from build123d import *

# Parameters (mm, degrees)
OUTER_START                              = 2.286
OUTER_CLAMP_LATCH_CUT_EXTRUDE5_DEPTH     = 2.794
OUTER_START_2                            = -1.143
OUTER_CLAMP_LATCH_CUT_EXTRUDE5_2_DEPTH   = 2.4129999
OUTER_START_3                            = -0.508
OUTER_CLAMP_LATCH_CUT_EXTRUDE5_3_OUTLI_R = 0.79375
OUTER_CLAMP_LATCH_CUT_EXTRUDE5_3_DEPTH   = 1.651
OUTER_START_4                            = 3.429
OUTER_CLAMP_LATCH_CUT_EXTRUDE5_4_OUTLI_R = 0.79375
OUTER_CLAMP_LATCH_CUT_EXTRUDE5_4_DEPTH   = 1.651
OUTER_START_5                            = 5.08
OUTER_CLAMP_LATCH_CUT_EXTRUDE5_5_DEPTH   = 1.27
OUTER_START_6                            = 1.2699999
OUTER_CLAMP_LATCH_CUT_EXTRUDE5_6_DEPTH   = 1.0160001
OUTER_START_7                            = -5.207
OUTER_CLAMP_LATCH_CUT_EXTRUDE5_7_OUTLI_R = 0.508
OUTER_CLAMP_LATCH_CUT_EXTRUDE5_7_DEPTH   = 2.54
SKETCH1_W                                = 0.762
SKETCH1_H                                = 1.524
CUT_EXTRUDE1_DEPTH                       = 14.441616644


with BuildPart() as part:
    # <Outer Clamp Latch>-<Cut-Extrude5>: read off the stored shape, not the designer's step
    # <Outer Clamp Latch>-<Cut-Extrude5> outline → <Outer Clamp Latch>-<Cut-Extrude5> (new body)
    with BuildSketch(Plane.XY.offset(OUTER_START)):
        Polygon((-4.699, -4.318), (-4.699, -2.667), (-6.596292399, -2.667), (-6.985, -3.340261314), (-6.985, -9.652), (-4.957886423, -9.652), (-3.937, -5.842), (-3.937, -4.318), align=None)
    extrude(amount=OUTER_CLAMP_LATCH_CUT_EXTRUDE5_DEPTH)

    # Outer Clamp Latch_-_Cut-Extrude5 4 outli → Outer Clamp Latch_-_Cut-Extrude5 4 (add)
    with BuildSketch(Plane.XY.offset(OUTER_START_4)):
        with BuildLine():
            Line((-4.699, -2.667), (-4.699, -2.6035))
            Line((-4.699, -2.6035), (-3.81, -2.6035))
            ThreePointArc((-3.81, -2.6035), (-2.435184671, -0.222249999), (-5.184815329, -0.22225))
            Line((-5.184815329, -0.22225), (-6.596292399, -2.667))
            Line((-6.596292399, -2.667), (-4.699, -2.667))
        make_face()
        with Locations((-3.81, -1.016)):
            Circle(OUTER_CLAMP_LATCH_CUT_EXTRUDE5_4_OUTLI_R, mode=Mode.SUBTRACT)
    extrude(amount=OUTER_CLAMP_LATCH_CUT_EXTRUDE5_4_DEPTH)

    # Outer Clamp Latch_-_Cut-Extrude5 5 outli → Outer Clamp Latch_-_Cut-Extrude5 5 (add)
    with BuildSketch(Plane.XY.offset(OUTER_START_5)):
        Polygon((-5.715, -3.340261314), (-6.985, -3.340261314), (-6.985, -9.652), (-5.715, -9.652), (-5.715, -5.207), align=None)
    extrude(amount=OUTER_CLAMP_LATCH_CUT_EXTRUDE5_5_DEPTH)



with BuildPart() as body_2:
    # Outer Clamp Latch_-_Cut-Extrude5 2 outli → Outer Clamp Latch_-_Cut-Extrude5 2 (new body)
    with BuildSketch(Plane.XY.offset(OUTER_START_2)):
        Polygon((-4.699, -4.318), (-4.699, -2.667), (-6.596292399, -2.667), (-6.985, -3.340261314), (-6.985, -9.652), (-4.957886423, -9.652), (-3.937, -5.842), (-3.937, -4.318), align=None)
    extrude(amount=OUTER_CLAMP_LATCH_CUT_EXTRUDE5_2_DEPTH)

    # Outer Clamp Latch_-_Cut-Extrude5 3 outli → Outer Clamp Latch_-_Cut-Extrude5 3 (add)
    with BuildSketch(Plane.XY.offset(OUTER_START_3)):
        with BuildLine():
            Line((-4.699, -2.667), (-4.699, -2.6035))
            Line((-4.699, -2.6035), (-3.81, -2.6035))
            ThreePointArc((-3.81, -2.6035), (-2.435184671, -0.222249999), (-5.184815329, -0.22225))
            Line((-5.184815329, -0.22225), (-6.596292399, -2.667))
            Line((-6.596292399, -2.667), (-4.699, -2.667))
        make_face()
        with Locations((-3.81, -1.016)):
            Circle(OUTER_CLAMP_LATCH_CUT_EXTRUDE5_3_OUTLI_R, mode=Mode.SUBTRACT)
    extrude(amount=OUTER_CLAMP_LATCH_CUT_EXTRUDE5_3_DEPTH)


with BuildPart() as part_1:
    add(part.part)

    add(body_2.part)  # Outer Clamp Latch_-_Cut-Extrude5 6 merges body 2
    # Outer Clamp Latch_-_Cut-Extrude5 6 outli → Outer Clamp Latch_-_Cut-Extrude5 6 (add)
    with BuildSketch(Plane.XY.offset(OUTER_START_6)):
        Polygon((-4.699, -4.318), (-4.699, -2.667), (-6.596292399, -2.667), (-6.985, -3.340261314), (-6.985, -9.652), (-4.957886423, -9.652), (-3.937, -5.842), (-3.937, -4.318), align=None)
    extrude(amount=OUTER_CLAMP_LATCH_CUT_EXTRUDE5_6_DEPTH)

    # Outer Clamp Latch_-_Cut-Extrude5 7 outli → Outer Clamp Latch_-_Cut-Extrude5 7 (cut)
    with BuildSketch(Plane(origin=(0, 0, 0), x_dir=(1, 0, 0), z_dir=(0, 1, 0)).offset(OUTER_START_7)):
        with Locations((-5.715, -1.778)):
            Circle(OUTER_CLAMP_LATCH_CUT_EXTRUDE5_7_OUTLI_R)
    extrude(amount=OUTER_CLAMP_LATCH_CUT_EXTRUDE5_7_DEPTH, mode=Mode.SUBTRACT)

    # Sketch1 → Cut-Extrude1 (cut, through all)
    with BuildSketch(Plane.XY.offset(5.08)):
        with Locations((-4.318, -5.08)):
            Rectangle(SKETCH1_W, SKETCH1_H)
    extrude(amount=-CUT_EXTRUDE1_DEPTH, mode=Mode.SUBTRACT)


solid = part_1.part
Verification items for the finished model (mm, model axes). A direction names the side the tool comes from. Give positions to 0.01 mm unless a question says otherwise; leave off trailing zeros. Write each loop counter-clockwise with the first axis right and the second up, starting at its lowest first coordinate (ties: lowest second). Pieces come first, ordered by that corner, then holes.
(1) Material ranges on line 1 (Z direction, x = -5.65, y = -2.25); line 2 (Y direction, x = -3.81, z = 3.95); line 3 (Z direction, x = -5, y = -3.75), recorded low to high.
(2) Cross-section at D-D (x = -4.4). Enter the section's corners in (y, z).
(3) Mould release check, pull along Z, two halves, no side actions. Record for faces 6 (the face through (-6, -6, 6.35)), 7 (the face through (-4, -2, 3.429)), 8 (the face through (-6.985, -6, 3)): +Z half, -Z half, draft (parallel to the pull), parting line (faces both ways), or undercut.
(4) Cross-section at B-B (x = -2.45). Enter the section's corners in (y, z), plus the area to 3 significant figures.
(5) Gauge pin test, flat ends, axial feed: pin 1 (2.5 mm diameter, centred on x = -4, y = -6.5, fed in from +Z); pin 2 (1.4 mm diameter, centred on x = -3.81, y = -1.016, fed in from +Z); pin 3 (1.5 mm diameter, centred on y = -1.5, z = 0.5, fed in from -X); pin 4 (2.5 mm diameter, centred on y = -4, z = 1.5, fed in from +X). Record the tip position at first contact, or that the pin passes through.
(6) Cross-section at C-C (z = 0). Enter the section's corners in (x, y) (1 decimal), plus the area to 3 significant figures.
(7) Access from +Z, -Z, +X, -X, +Y, -Y to the whole of each face (thin tool, end or side, straight path). Record for faces 1 (the face through (-5.7, -5.207, 1.8)), 2 (the face through (-4, -2, -0.508)), 3 (the face through (-5.715, -7, 6)), 4 (the face through (-4, -2.604, 4)), 5 (the face through (-6, -2.667, 3)).
(8) Cross-section at A-A (z = 2.75). Enter the section's corners in (x, y) (3 decimals), plus the area to 3 significant figures.
Worked out:
1. line 1: z = -0.51 to 1.14, 3.43 to 5.08
1. line 2: y = -2.6 to -1.81, -0.22 to 0.57
1. line 3: z = -1.14 to 5.08
2. outline: (-7.57, -1.14) - (-5.84, -1.14) - (-5.84, 5.08) - (-7.57, 5.08) - close; (-2.6, -0.51) - (-1.55, -0.51) - (-1.55, 1.14) - (-2.6, 1.14) - close; (-2.6, 3.43) - (-1.55, 3.43) - (-1.55, 5.08) - (-2.6, 5.08) - close; (-0.49, -0.51) - (0.46, -0.51) - (0.46, 1.14) - (-0.49, 1.14) - close; (-0.49, 3.43) - (0.46, 3.43) - (0.46, 5.08) - (-0.49, 5.08) - close
3. face 6: +Z half
3. face 7: undercut
3. face 8: draft
4. outline: (-1.83, -0.51) - (-0.2, -0.51) - (-0.2, 1.14) - (-1.83, 1.14) - close; (-1.83, 3.43) - (-0.2, 3.43) - (-0.2, 5.08) - (-1.83, 5.08) - close
4. area: 5.41 mm2
5. pin 1: stops at z = 5.08
5. pin 2: passes through
5. pin 3: stops at x = -6.36
5. pin 4: stops at x = -4.7
6. outline: (-7, -9.7) - (-5, -9.7) - (-3.9, -5.8) - (-4.7, -5.8) - (-4.7, -2.6) - (-3.8, -2.6) arc R1.6 ccw (long way) to (-5.2, -0.2) - (-7, -3.3) - close; hole circle Ø1.6 at (-3.8, -1)
6. area: 24.6 mm2
7. face 1: +Y
7. face 2: -Z, +X, -X, +Y
7. face 3: +Z, +X, +Y, -Y
7. face 4: +Z, -Z, +X
7. face 5: +X, -X, +Y
8. outline: (-6.985, -9.652) - (-4.958, -9.652) - (-3.937, -5.842) - (-4.699, -5.842) - (-4.699, -2.667) - (-6.596, -2.667) - (-6.985, -3.34) - close
8. area: 16.8 mm2
